Source: CAD feature listing. Evaluate the final solid. Frame: model axes, mm. A direction names the side the tool comes from. Coordinates: 2 decimals unless noted, no trailing zeros. Order: outer loops, then holes, each group sorted by start corner. A loop starts at its lowest first (then second) coordinate and runs counter-clockwise, first axis right, second up. Notation, with made-up numbers: (8.5, -0.75) - (22.5, -0.75) arc R19 ccw to (22.5, 17.25) - close; hole circle Ø8 at (39, -34.75). An arc over 180 degrees is marked (long way). One line per question, with ' | ' between items. Start each with the question number.
(1) Draft query along Y for faces 3 (the cylindrical face through (-0.54, -2.44, 2.99)), 4 (the flat face through (-9, 0, 2)), 5 (the flat face through (-7.947, 2.705, 0.986)), 6 (the flat face through (-7.746, -2.725, 0.986)). Return one class per face: +Y half, -Y half, draft (parallel to the pull), parting line (faces both ways), or undercut.
(2) Section A-A (x = 0). Return the cut outline in (y, z).
(3) Section D-D (z = 2.3). Return the cut outline in (x, y).
(4) Section C-C (z = 0.65). Return the cut outline in (x, y), then the cut area to 4 significant figures.
(5) Access query for faces 1 (the flat face through (-7, 0, 0)), 2 (the flat face through (-1, 1, 2)). Directions: +Z, -Z, +X, -X, +Y, -Y. A direction counts if a zero-diameter tool reaches every point of the face in a straight line with its end or side. Return the directions, or none.
(6) Contact query for flat-ended pins moving along their axis: P1, Ø2.5, axis at x = -15, y = 0, coming from the +Z side; P2, Ø1, axis at x = -14.5, y = -2.5, coming from the -Z side. Output: stop coordinate, or through.
(7) Line query: line 1 along Y through (x, z) = (0, 1); line 2 along Y through (x, z) = (0, 2.8); line 3 along Z through (x, y) = (-7.5, -0.25). Output: solid intervals per line, ascending.
(8) Section B-B (y = 0). Return the cut outline in (x, z).
from build123d import *

# Parameters (mm, degrees)
SKETCH1_R           = 3.5
SKETCH1_R_2         = 2.5
BOSS_EXTRUDE1_DEPTH = 4
SKETCH2_R           = 1
BOSS_EXTRUDE2_DEPTH = 2
SKETCH3_R           = 2.5
SKETCH3_R_2         = 1.25
BOSS_EXTRUDE3_DEPTH = 2


with BuildPart() as part:
    # Sketch1 → Boss-Extrude1 (new body)
    with BuildSketch(Plane.XY):
        Circle(SKETCH1_R)
        Circle(SKETCH1_R_2, mode=Mode.SUBTRACT)
    extrude(amount=BOSS_EXTRUDE1_DEPTH)

    # Sketch2 → Boss-Extrude2 (add)
    with BuildSketch(Plane(origin=(0, 0, 0), x_dir=(-1, 0, 0), z_dir=(0, 0, -1))):
        with BuildLine():
            Line((15, 2), (0.693069307, 3.430693069))
            ThreePointArc((0.693069307, 3.430693069), (2.708850547, 2.216332266), (3.5, 0))
            ThreePointArc((3.5, 0), (2.708850547, -2.216332266), (0.693069307, -3.430693069))
            Line((0.693069307, -3.430693069), (15, -2))
            ThreePointArc((15, -2), (17, 0), (15, 2))
        make_face()
        with Locations((15, 0)):
            Circle(SKETCH2_R, mode=Mode.SUBTRACT)
    extrude(amount=-BOSS_EXTRUDE2_DEPTH)

    # Sketch3 → Boss-Extrude3 (add)
    with BuildSketch(Plane(origin=(0, 0, 0), x_dir=(-1, 0, 0), z_dir=(0, 0, -1))):
        Circle(SKETCH3_R)
        Circle(SKETCH3_R_2, mode=Mode.SUBTRACT)
    extrude(amount=-BOSS_EXTRUDE3_DEPTH)


solid = part.part
Response values:
1) face 3: undercut | face 4: draft | face 5: +Y half | face 6: -Y half
2) outline: (-3.5, 0) - (-1.25, 0) - (-1.25, 2) - (-2.5, 2) - (-2.5, 4) - (-3.5, 4) - close; (1.25, 0) - (3.5, 0) - (3.5, 4) - (2.5, 4) - (2.5, 2) - (1.25, 2) - close
3) outline: circle Ø7 at (0, 0); hole circle Ø5 at (0, 0)
4) outline: (-15, -2) - (-0.69, -3.43) arc R3.5 ccw (long way) to (-0.69, 3.43) - (-15, 2) arc R2 ccw to start; hole circle Ø2 at (-15, 0); hole circle Ø2.5 at (0, 0) | area: 100.0 mm²
5) face 1: -Z, +X, -X, +Y, -Y | face 2: +Z
6) P1: stops at z = 2 | P2: stops at z = 0
7) line 1: y = -3.5 to -1.25, 1.25 to 3.5 | line 2: y = -3.5 to -2.5, 2.5 to 3.5 | line 3: z = 0 to 2
8) outline: (-17, 0) - (-16, 0) - (-16, 2) - (-17, 2) - close; (-14, 0) - (-1.25, 0) - (-1.25, 2) - (-2.5, 2) - (-2.5, 4) - (-3.5, 4) - (-3.5, 2) - (-14, 2) - close; (1.25, 0) - (3.5, 0) - (3.5, 4) - (2.5, 4) - (2.5, 2) - (1.25, 2) - close
